Geometry: final body of the model. Coordinates: model frame, mm. A direction names the side the tool comes from. Round coordinates to 2 decimals unless told otherwise and drop trailing zeros. Loops run counter-clockwise (first coordinate to the right, second up) from the corner with the lowest first, then second, coordinate; pieces in that order, holes last. Notation, with made-up numbers: M 17,27.25 L 36,27.25 A27 cw 36,63.25 Z; hole C 52,0 d6. An arc over 180 degrees is marked long. Return JSON: item names as keys, results as strings.
Solid Edge part; units mm, degrees
sketch "Sketch1" plane through (0, 0, 0) normal (1, 0, 0) x (0, 1, 0)
  line L0 (0, 0) -> (3, 0)
  line L1 (3, 0) -> (3, -146.2)
  line L2 (3, -146.2) -> (8, -146.2)
  line L3 (8, -146.2) -> (8, -151.5333)
  line L4 (8, -151.5333) -> (0, -151.5333)
  line L5 (0, -151.5333) -> (0, 0)
revolve "RevolvedProtrusion1" add sketch "Sketch1" angle 360 about axis through (0, 0, -151.5333) along (0, 0, 1)
sketch "Sketch2" plane through (0, 0, 0) normal (1, 0, 0) x (0, 1, 0)
  line L0 (5, 2) -> (-5, 2)
  line L1 (-5, 2) -> (-5, -4.4434)
  line L2 (-5, -4.4434) -> (-2.5, -3)
  line L3 (-2.5, -3) -> (-2.5, 0)
  line L4 (-2.5, 0) -> (2.5, 0)
  line L5 (2.5, 0) -> (2.5, -3)
  line L6 (2.5, -3) -> (5, -4.4434)
  line L7 (5, -4.4434) -> (5, 2)
extrude "ExtrudedCutout_1" cut sketch "Sketch2" against normal blind 3 and the other way blind 3
sketch "Sketch3" plane through (0, 0, 0) normal (1, 0, 0) x (0, 1, 0)
  line L0 (0, 16) -> (2.3865, 16)
  line L1 (2.3865, 16) -> (3, 15.3865)
  line L2 (3, 15.3865) -> (3, 0.6135)
  line L3 (3, 0.6135) -> (2.3865, 0)
  line L4 (2.3865, 0) -> (0, 0)
  line L5 (0, 0) -> (0, 16)
revolve "RevolvedProtrusion2" add sketch "Sketch3" angle 360 about axis through (0, 0, 0) along (0, 0, 1)
properties part number "BumbleB0479"
Q1. Reachability of faces 1 (the flat face through (0, -2.5, -2)), 2 (the flat face through (-0.1, 3.4, -146.2)), 3 (the flat face through (0, 2.5, -1)) from +Z, -Z, +X, -X, +Y, -Y: full face, straight path, thin tool, end or side. Return the list, or none.
Determined:
{"face 1": "+X, -X, -Y", "face 2": "+Z", "face 3": "+X, -X, +Y"}
Q2. Section query C-C (x = 5). Output: boundary loops of the cut face in (y, z) (3 decimals), plus the area to 3 significant figures.
Determined:
{"outline": "M -6.245,-151.533 L 6.245,-151.533 L 6.245,-146.2 L -6.245,-146.2 Z", "area": "66.6 mm^2"}
Q3. Pin query (flat end, axial travel): pin 1 (1.5 mm diameter, centred on x = 0, z = -1, fed in from +Y); pin 2 (5 mm diameter, centred on x = -3.5, y = 6.5, fed in from +Z); pin 3 (0.9 mm diameter, centred on x = -0.5, z = -1.5, fed in from -Y). Return the tip coordinate at first contact, or that it passes through.
Determined:
{"pin 1": "stops at y = 2.5", "pin 2": "stops at z = -146.2", "pin 3": "stops at y = -2.5"}
Q4. Material intervals for L1, parallel to Z at x = -2.25, y = 2.75; L2, parallel to Y at x = 0.25, z = -104.5; L3, parallel to Y at x = -2.5, z = -53.5, sorted ascending.
Determined:
{"L1": "z = -151.53 to -146.2", "L2": "y = -2.99 to 2.99", "L3": "y = -1.66 to 1.66"}
Q5. Section query A-A (y = 0). Output: boundary loops of the cut face in (x, z), plus the area to 3 significant figures.
Determined:
{"outline": "M -8,-151.53 L 8,-151.53 L 8,-146.2 L 3,-146.2 L 3,0 L 2.39,0 L 3,0.61 L 3,15.39 L 2.39,16 L -2.39,16 L -3,15.39 L -3,0.61 L -2.39,0 L -3,0 L -3,-146.2 L -8,-146.2 Z", "area": "1,060 mm^2"}
Q6. Section query B-B (z = -71). Output: boundary loops of the cut face in (x, y), plus the area to 3 significant figures.
Determined:
{"outline": "C 0,0 d6", "area": "28.3 mm^2"}
